Check sheet for the modelled part. Datum: model origin and axes. Units: mm. Face numbers are marked on the shaded views. A direction names the side the tool comes from. Round coordinates to 2 decimals unless told otherwise and drop trailing zeros. Write each loop counter-clockwise with the first axis right and the second up, starting at its lowest first coordinate (ties: lowest second). Pieces come first, ordered by that corner, then holes. Notation, with made-up numbers: M 29.5,27 L 44.5,27 A18 cw 44.5,42 Z; hole C 58.25,47 d3. An arc over 180 degrees is marked long. Answer in a Markdown table with one row per item.
```python
from build123d import *

# Parameters (mm, degrees)
SKETCH_3_R           = 48
EXTRUDE_2_DEPTH      = 3
SKETCH_4_R           = 3
CUT_EXTRUDE_1_DEPTH  = 3
EXTRUDE_3_DEPTH      = 35
SKETCH_6_R           = 3
SKETCH_6_R_2         = 1.5
CUT_EXTRUDE_2_DEPTH  = 35
SKETCH_7_R           = 1.55
CUT_EXTRUDE_5_DEPTH  = 35
SKETCH_8_R           = 2.05
CUT_EXTRUDE_6_DEPTH  = 10
SKETCH_9_R           = 1.55
CUT_EXTRUDE_7_DEPTH  = 10
SKETCH_10_W          = 35
SKETCH_10_H          = 25
EXTRUDE_4_DEPTH      = 2
SKETCH_11_R          = 3
SKETCH_11_R_2        = 1.5
CUT_EXTRUDE_8_DEPTH  = 2
EXTRUDE_START        = -3
SKETCH_12_R          = 49
SKETCH_12_R_2        = 48
EXTRUDE_5_DEPTH      = 3
SKETCH_14_R          = 51
SKETCH_14_R_2        = 49
EXTRUDE_6_DEPTH      = 65
SKETCH_15_R          = 51
SKETCH_15_R_2        = 49
EXTRUDE_7_DEPTH      = 3
SKETCH_16_R          = 60
SKETCH_16_R_2        = 51
EXTRUDE_9_DEPTH      = 3
SKETCH_19_W          = 65
SKETCH_19_H          = 33.883358742
CUT_EXTRUDE_9_DEPTH  = 135.996296245
SKETCH_21_W          = 65
SKETCH_21_H          = 33.883358742
CUT_EXTRUDE_10_DEPTH = 110.854449159


with BuildPart() as part:
    # Sketch 3 → Extrude 2 (new body)
    with BuildSketch(Plane.XY):
        Circle(SKETCH_3_R)
    extrude(amount=EXTRUDE_2_DEPTH)

    # Sketch 4 → Cut-Extrude 1 (cut)
    with BuildSketch(Plane.XY.offset(3)):
        Circle(SKETCH_4_R)
    extrude(amount=-CUT_EXTRUDE_1_DEPTH, mode=Mode.SUBTRACT)

    # Sketch 5 → Extrude 3 (add)
    with BuildSketch(Plane.XY.offset(3)):
        with BuildLine():
            ThreePointArc((0, 12.5), (0.146446609, 12.853553391), (0.5, 13))
            Line((0.5, 13), (39.5, 13))
            ThreePointArc((39.5, 13), (39.853553391, 12.853553391), (40, 12.5))
            Line((40, 12.5), (40, -12.5))
            ThreePointArc((40, -12.5), (39.853553391, -12.853553391), (39.5, -13))
            Line((39.5, -13), (0.5, -13))
            ThreePointArc((0.5, -13), (0.146446609, -12.853553391), (0, -12.5))
            Line((0, -12.5), (0, -11.5))
            ThreePointArc((0, -11.5), (0.146446609, -11.146446609), (0.5, -11))
            Line((0.5, -11), (37.5, -11))
            ThreePointArc((37.5, -11), (37.853553391, -10.853553391), (38, -10.5))
            Line((38, -10.5), (38, 0))
            Line((38, 0), (38, 10.5))
            ThreePointArc((38, 10.5), (37.853553391, 10.853553391), (37.5, 11))
            Line((37.5, 11), (0.5, 11))
            ThreePointArc((0.5, 11), (0.146446609, 11.146446609), (0, 11.5))
            Line((0, 11.5), (0, 12.5))
        make_face()
    extrude(amount=EXTRUDE_3_DEPTH)

    # Sketch 6 → Cut-Extrude 2 (cut)
    with BuildSketch(Plane(origin=(40, 0, 0), x_dir=(0, 0, -1), z_dir=(1, 0, 0))):
        with Locations((-25, 0)):
            Circle(SKETCH_6_R)
        with Locations((-20, -5)):
            Circle(SKETCH_6_R_2)
        with Locations((-20, 5)):
            Circle(SKETCH_6_R_2)
        with Locations((-30, -5)):
            Circle(SKETCH_6_R_2)
        with Locations((-30, 5)):
            Circle(SKETCH_6_R_2)
    extrude(amount=-CUT_EXTRUDE_2_DEPTH, mode=Mode.SUBTRACT)

    # Sketch 7 → Cut-Extrude 5 (cut)
    with BuildSketch(Plane.XY.offset(3)):
        with Locations((-35, 0)):
            Circle(SKETCH_7_R)
        with Locations((-24.748737342, 24.748737342)):
            Circle(SKETCH_7_R)
        with Locations((0, 35)):
            Circle(SKETCH_7_R)
        with Locations((24.748737342, 24.748737342)):
            Circle(SKETCH_7_R)
        with Locations((35, 0)):
            Circle(SKETCH_7_R)
        with Locations((24.748737342, -24.748737342)):
            Circle(SKETCH_7_R)
        with Locations((0, -35)):
            Circle(SKETCH_7_R)
        with Locations((-24.748737342, -24.748737342)):
            Circle(SKETCH_7_R)
    extrude(amount=-CUT_EXTRUDE_5_DEPTH, mode=Mode.SUBTRACT)

    # Sketch 8 → Cut-Extrude 6 (cut)
    with BuildSketch(Plane.XY.offset(3)):
        with Locations((0, 35)):
            Circle(SKETCH_8_R)
        with Locations((24.748737342, 24.748737342)):
            Circle(SKETCH_8_R)
        with Locations((35, 0)):
            Circle(SKETCH_8_R)
        with Locations((24.748737342, -24.748737342)):
            Circle(SKETCH_8_R)
        with Locations((0, -35)):
            Circle(SKETCH_8_R)
        with Locations((-24.748737342, -24.748737342)):
            Circle(SKETCH_8_R)
        with Locations((-35, 0)):
            Circle(SKETCH_8_R)
        with Locations((-24.748737342, 24.748737342)):
            Circle(SKETCH_8_R)
    extrude(amount=-CUT_EXTRUDE_6_DEPTH, mode=Mode.SUBTRACT)

    # Sketch 9 → Cut-Extrude 7 (cut)
    with BuildSketch(Plane.XY.offset(3)):
        with Locations((-5, 5)):
            Circle(SKETCH_9_R)
        with Locations((5, 5)):
            Circle(SKETCH_9_R)
        with Locations((5, -5)):
            Circle(SKETCH_9_R)
        with Locations((-5, -5)):
            Circle(SKETCH_9_R)
    extrude(amount=-CUT_EXTRUDE_7_DEPTH, mode=Mode.SUBTRACT)

    # Sketch 10 → Extrude 4 (add)
    with BuildSketch(Plane(origin=(40, 0, 0), x_dir=(0, 0, -1), z_dir=(1, 0, 0))):
        with Locations((-20.5, 0)):
            Rectangle(SKETCH_10_W, SKETCH_10_H)
    extrude(amount=-EXTRUDE_4_DEPTH)

    # Sketch 11 → Cut-Extrude 8 (cut)
    with BuildSketch(Plane(origin=(40, 0, 0), x_dir=(0, 0, -1), z_dir=(1, 0, 0))):
        with Locations((-28, 0)):
            Circle(SKETCH_11_R)
        with Locations((-33, 5)):
            Circle(SKETCH_11_R_2)
        with Locations((-28, 7.071067812)):
            Circle(SKETCH_11_R_2)
        with Locations((-23, 5)):
            Circle(SKETCH_11_R_2)
        with Locations((-20.928932188, 0)):
            Circle(SKETCH_11_R_2)
        with Locations((-23, -5)):
            Circle(SKETCH_11_R_2)
        with Locations((-28, -7.071067812)):
            Circle(SKETCH_11_R_2)
        with Locations((-33, -5)):
            Circle(SKETCH_11_R_2)
        with Locations((-35.071067812, 0)):
            Circle(SKETCH_11_R_2)
    extrude(amount=-CUT_EXTRUDE_8_DEPTH, mode=Mode.SUBTRACT)

    # Sketch 12 → Extrude 5 (add)
    with BuildSketch(Plane.XY.offset(3).offset(EXTRUDE_START)):
        Circle(SKETCH_12_R)
        Circle(SKETCH_12_R_2, mode=Mode.SUBTRACT)
    extrude(amount=EXTRUDE_5_DEPTH)



with BuildPart() as body_2:
    # Sketch 14 → Extrude 6 (new body)
    with BuildSketch(Plane.XY.offset(3)):
        Circle(SKETCH_14_R)
        Circle(SKETCH_14_R_2, mode=Mode.SUBTRACT)
    extrude(amount=EXTRUDE_6_DEPTH)


with BuildPart() as part_1:
    add(part.part)

    add(body_2.part)  # Extrude 7 merges body 2
    # Sketch 15 → Extrude 7 (add)
    with BuildSketch(Plane(origin=(0, 0, 0), x_dir=(-1, 0, 0), z_dir=(0, 0, -1))):
        Circle(SKETCH_15_R)
        with Locations(Location((0, 0, 0), (0, 0, 180))):
            Circle(SKETCH_15_R_2, mode=Mode.SUBTRACT)
    extrude(amount=-EXTRUDE_7_DEPTH)

    # Sketch 16 → Extrude 9 (add)
    with BuildSketch(Plane(origin=(0, 0, 0), x_dir=(-1, 0, 0), z_dir=(0, 0, -1))):
        Circle(SKETCH_16_R)
        Circle(SKETCH_16_R_2, mode=Mode.SUBTRACT)
    extrude(amount=-EXTRUDE_9_DEPTH)

    # Sketch 19 → Cut-Extrude 9 (cut, through all)
    with BuildSketch(Plane(origin=(40, 0, 0), x_dir=(0, 0, -1), z_dir=(1, 0, 0))):
        with Locations((-35.5, 0.112944529)):
            Rectangle(SKETCH_19_W, SKETCH_19_H)
    extrude(amount=CUT_EXTRUDE_9_DEPTH, mode=Mode.SUBTRACT)

    # Sketch 21 → Cut-Extrude 10 (cut, through all)
    with BuildSketch(Plane.ZY.offset(2)):
        with Locations((35.5, 0.112944529)):
            Rectangle(SKETCH_21_W, SKETCH_21_H)
    extrude(amount=CUT_EXTRUDE_10_DEPTH, mode=Mode.SUBTRACT)


solid = part_1.part
```
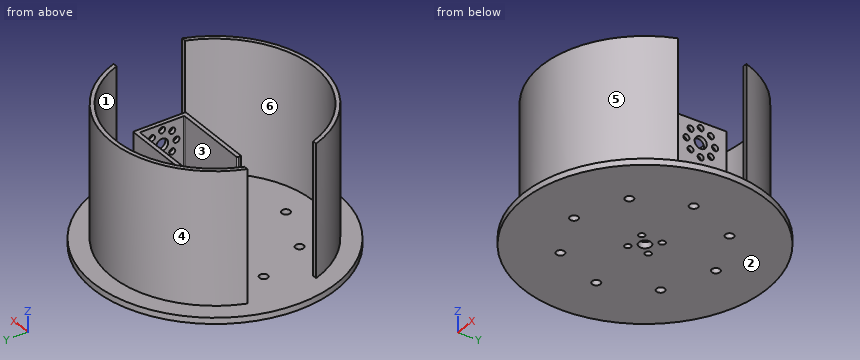
1. Access from +Z, -Z, +X, -X, +Y, -Y to the whole of each face (thin tool, end or side, straight path). Record for the marked faces 5 and 6.
Found:
| item | result |
|---|---|
| face 5 | +Z, -Y |
| face 6 | +Z |
2. Go/stop test with flat-tipped pins: pin 1 (23 mm diameter, centred on y = 3, z = 28.5, fed in from -X); pin 2 (2.5 mm diameter, centred on x = -5, y = 5, fed in from -Z); pin 3 (1.1 mm diameter, centred on x = 46.5, z = 33.5, fed in from +Y); pin 4 (5 mm diameter, centred on x = 10.5, z = 60, fed in from +Y). Record where each tip stops, or that it passes through.
Found:
| item | result |
|---|---|
| pin 1 | stops at x = 0 |
| pin 2 | passes through |
| pin 3 | stops at y = 22.13 |
| pin 4 | stops at y = 50.37 |
3. Section check B-B, the plane x = 5. Record the cut outline in (y, z).
Found:
| item | result |
|---|---|
| outline | M -59.79,0 L -6.55,0 L -6.55,3 L -11,3 L -11,38 L -13,38 L -13,3 L -48.74,3 L -48.74,68 L -50.75,68 L -50.75,3 L -59.79,3 Z; M -3.45,0 L 3.45,0 L 3.45,3 L -3.45,3 Z; M 6.55,0 L 59.79,0 L 59.79,3 L 50.75,3 L 50.75,68 L 48.74,68 L 48.74,3 L 13,3 L 13,38 L 11,38 L 11,3 L 6.55,3 Z |
4. Section check D-D, the plane y = -35. Record the cut outline in (x, z), and give its area (3 significant figures).
Found:
| item | result |
|---|---|
| outline | M -48.73,0 L -2.05,0 L -2.05,3 L -34.29,3 L -34.29,68 L -37.09,68 L -37.09,3 L -48.73,3 Z; M 2.05,0 L 48.73,0 L 48.73,3 L 37.09,3 L 37.09,68 L 34.29,68 L 34.29,3 L 2.05,3 Z |
| area | 644 mm2 |
5. Section check C-C, the plane z = 45. Record the cut outline in (x, y).
Found:
| item | result |
|---|---|
| outline | M -48.14,-16.83 A51 ccw 48.14,-16.83 L 46.02,-16.83 A49 cw -46.02,-16.83 Z; M -48.06,17.05 L -45.94,17.05 A49 cw 45.94,17.05 L 48.06,17.05 A51 ccw Z |
6. Draft check along Y on the marked faces 1, 2, 3 and 4. Enter one of: +Y half, -Y half, draft (parallel to the pull), parting line (faces both ways), or undercut.
Found:
| item | result |
|---|---|
| face 1 | undercut |
| face 2 | draft |
| face 3 | undercut |
| face 4 | +Y half |
7. Section check A-A, the plane z = 16. Record the cut outline in (x, y).
Found:
| item | result |
|---|---|
| outline | M -48.14,-16.83 A51 ccw 48.14,-16.83 L 46.02,-16.83 A49 cw -46.02,-16.83 Z; M -48.06,17.05 L -45.94,17.05 A49 cw 45.94,17.05 L 48.06,17.05 A51 ccw Z; M 0,-12.5 A0.5 ccw 0.5,-13 L 39.5,-13 A0.5 ccw 40,-12.5 L 40,12.5 A0.5 ccw 39.5,13 L 0.5,13 A0.5 ccw 0,12.5 L 0,11.5 A0.5 ccw 0.5,11 L 37.5,11 A0.5 cw 38,10.5 L 38,-10.5 A0.5 cw 37.5,-11 L 0.5,-11 A0.5 ccw 0,-11.5 Z |
8. Scan lines: L1, parallel to Y at x = 0.5, z = 40; L2, parallel to Y at x = 5, z = 2.35; L3, parallel to Z at x = -8, y = 29. Record each from-to range of solid material in increasing order.
Found:
| item | result |
|---|---|
| L1 | y = -51 to -49, 49 to 51 |
| L2 | y = -59.79 to -6.55, -3.45 to 3.45, 6.55 to 59.79 |
| L3 | z = 0 to 3 |
